Geometry: final body of the model. Coordinates: model frame, mm. Face numbers are marked on the shaded views. A direction names the side the tool comes from. Give positions to 0.01 mm unless a question says otherwise; leave off trailing zeros. Order: outer loops, then holes, each group sorted by start corner. A loop starts at its lowest first (then second) coordinate and runs counter-clockwise, first axis right, second up. Notation, with made-up numbers: (-37.75, 72) - (8.25, 72) arc R29 ccw to (8.25, 98) - close; hole circle Ø11 at (12.25, 2.5). An arc over 180 degrees is marked (long way). Put each result on its own line as item: value. Start each with the question number.
1. Mould query, pull axis X, two halves, no side actions, for the marked faces 3, 4 and 5. Classes: pulls with the +X half, pulls with the -X half, needs draft (parallel to the pull), parting line crosses it, or undercut.
2. Section A-A on x = 3. Return the cut outline in (y, z), plus the area to 3 significant figures.
3. Section D-D on x = -8.25. Return the cut outline in (y, z), plus the area to 3 significant figures.
4. First-contact query: P1, Ø2, axis at x = -5, z = 0, coming from the +Y side; P2, Ø1.6, axis at y = 0.5, z = -2.5, coming from the -X side; P3, Ø0.6, axis at y = 0.5, z = -4, coming from the +X side; P4, Ø1.3, axis at x = -6, z = 1.5, coming from the -Y side. Flat tips, straight axial feed; report the tip coordinate or a pass-through.
5. Ray query, line 1 along Z through (x, y) = (-5, 0.5); line 2 along Y through (x, z) = (3, 4); line 3 along Z through (x, y) = (3.5, 4). Return the intervals inside material, ascending. Write a range as from..to.
6. Set-up query: the marked faces 1 and 2. Return all of +Z, -Z, +X, -X, +Y, -Y with unobstructed straight access to the full face (end or side cutting, diameter ignored); none if empty.
7. Section B-B on z = -5.25. Return the cut outline in (x, y).
8. Section C-C on y = 1.75. Return the cut outline in (x, z).
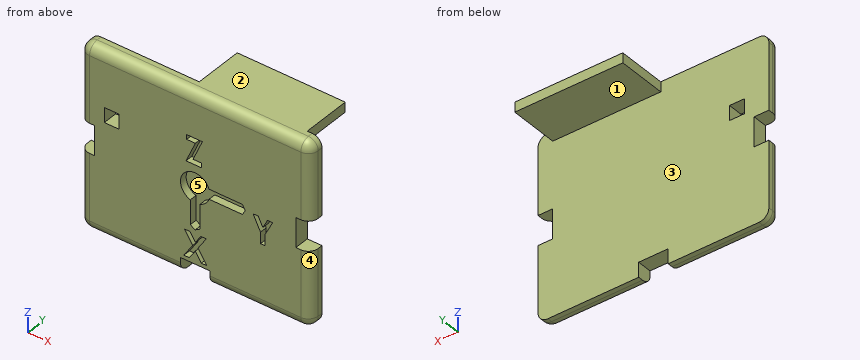
from build123d import *

# Parameters (mm, degrees)
SKETCH1_W           = 23.5
SKETCH1_H           = 18.5
BOSS_EXTRUDE1_DEPTH = 1.5
SKETCH2_W           = 3
SKETCH2_H           = 1.5
SKETCH2_W_2         = 1.5
SKETCH2_H_2         = 3
CUT_EXTRUDE1_DEPTH  = 1.5
SKETCH3_W           = 10
SKETCH3_H           = 1
BOSS_EXTRUDE2_DEPTH = 5
CUT_EXTRUDE3_DEPTH  = 0.75
SKETCH5_W           = 1.5
SKETCH5_H           = 1.5
CUT_EXTRUDE4_DEPTH  = 1.5
FILLET1_R           = 1
FILLET4_R           = 1
SKETCH7_W           = 0.998185699
SKETCH7_H           = 1
BOSS_EXTRUDE3_DEPTH = 5


with BuildPart() as part:
    # Sketch1 → Boss-Extrude1 (new body)
    with BuildSketch(Plane(origin=(0, 0, 0), x_dir=(1, 0, 0), z_dir=(0, 1, 0))):
        with Locations((-5.985849057, 1.668632075)):
            Rectangle(SKETCH1_W, SKETCH1_H)
    extrude(amount=BOSS_EXTRUDE1_DEPTH)

    # Sketch2 → Cut-Extrude1 (cut)
    with BuildSketch(Plane(origin=(0, 1.5, 0), x_dir=(1, 0, 0), z_dir=(0, 1, 0))):
        with Locations((-5.985849057, 10.168632075)):
            Rectangle(SKETCH2_W, SKETCH2_H)
        with Locations((-16.985849057, 1.668632075)):
            Rectangle(SKETCH2_W_2, SKETCH2_H_2)
        with Locations((5.014150943, 1.668632075)):
            Rectangle(SKETCH2_W_2, SKETCH2_H_2)
    extrude(amount=-CUT_EXTRUDE1_DEPTH, mode=Mode.SUBTRACT)

    # Sketch3 → Boss-Extrude2 (add)
    with BuildSketch(Plane(origin=(0, 1.5, 0), x_dir=(1, 0, 0), z_dir=(0, 1, 0))):
        with Locations((-0.735849057, -7.081367925)):
            Rectangle(SKETCH3_W, SKETCH3_H)
    extrude(amount=BOSS_EXTRUDE2_DEPTH)

    # Sketch4 → Cut-Extrude3 (cut)
    with BuildSketch(Plane.XZ):
        with BuildLine():
            Line((-1.177314548, -2.300719994), (-0.888639414, -1.800719994))
            Line((-0.888639414, -1.800719994), (-1.177314548, -1.300719994))
            Line((-1.177314548, -1.300719994), (-4.571635494, -1.300719994))
            ThreePointArc((-4.571635494, -1.300719994), (-7.046509228, -0.740059822), (-6.485849057, -3.214933557))
            Line((-6.485849057, -3.214933557), (-6.485849057, -5.700361827))
            Line((-6.485849057, -5.700361827), (-5.985849057, -5.989036962))
            Line((-5.985849057, -5.989036962), (-5.485849057, -5.700361827))
            Line((-5.485849057, -5.700361827), (-5.485849057, -3.214933557))
            ThreePointArc((-5.485849057, -3.214933557), (-4.925188885, -2.861380166), (-4.571635494, -2.300719994))
            Line((-4.571635494, -2.300719994), (-1.177314548, -2.300719994))
        make_face()
        Polygon((-7.080591406, -6.388557959), (-6.520895893, -6.388557959), (-5.968090572, -7.238171507), (-5.41422522, -6.388557959), (-4.853999693, -6.388557959), (-5.688242815, -7.668013421), (-4.798878165, -9.034391292), (-5.358573678, -9.034391292), (-5.968090572, -8.09732532), (-6.579197509, -9.034391292), (-7.139423037, -9.034391292), (-6.247938328, -7.667483406), align=None)
        Polygon((-6.848224631, 3.131460083), (-5.253940443, 3.131460083), (-6.201606709, 0.960519912), (-5.321782324, 0.960519912), (-5.321782324, 0.48562675), (-6.916066512, 0.48562675), (-5.967870231, 2.656566921), (-6.848224631, 2.656566921), align=None)
        Polygon((-0.096157656, -1.744646719), (0.43226699, -1.744646719), (0.904510079, -2.672702441), (1.376753168, -1.744646719), (1.905177814, -1.744646719), (1.14195666, -3.244588292), (1.14195666, -4.390480052), (0.667063498, -4.390480052), (0.667063498, -3.244588292), align=None)
    extrude(amount=-CUT_EXTRUDE3_DEPTH, mode=Mode.SUBTRACT)

    # Sketch5 → Cut-Extrude4 (cut)
    with BuildSketch(Plane.XZ):
        with Locations((-14.485849057, 1.331367925)):
            Rectangle(SKETCH5_W, SKETCH5_H)
    extrude(amount=-CUT_EXTRUDE4_DEPTH, mode=Mode.SUBTRACT)

    # Fillet1
    fillet1_edges = [part.edges().sort_by_distance(p)[0] for p in [
        (-12.610849057, 0, -10.918632075),
        (5.764150943, 0, -7.043632075),
        (0.639150943, 0, -10.918632075),
        (-17.735849057, 0, -7.043632075),
        (-17.735849057, 0.75, -10.918632075),
        (5.764150943, 0.75, -10.918632075),
    ]]
    fillet(fillet1_edges, radius=FILLET1_R)

    # Fillet4
    fillet4_edges = [part.edges().sort_by_distance(p)[0] for p in [
        (-17.735849057, 0, 3.706367925),
        (5.764150943, 0, 3.706367925),
        (-5.985849057, 0, 7.581367925),
        (5.764150943, 0.75, 7.581367925),
        (-17.735849057, 0.75, 7.581367925),
    ]]
    fillet(fillet4_edges, radius=FILLET4_R)

    # Sketch7 → Boss-Extrude3 (add)
    with BuildSketch(Plane(origin=(0, 1.5, 0), x_dir=(1, 0, 0), z_dir=(0, 1, 0))):
        with Locations((-6.234941907, -7.081367925)):
            Rectangle(SKETCH7_W, SKETCH7_H)
    extrude(amount=BOSS_EXTRUDE3_DEPTH)


solid = part.part
Resolved:
1. face 3: needs draft
1. face 4: pulls with the +X half
1. face 5: undercut
2. outline: (0, -9.92) arc R1 ccw to (1, -10.92) - (1.5, -10.92) - (1.5, 6.58) - (6.5, 6.58) - (6.5, 7.58) - (1, 7.58) arc R1 ccw to (0, 6.58) - close
2. area: 32.3 mm^2
3. outline: (0, -9.92) arc R1 ccw to (1, -10.92) - (1.5, -10.92) - (1.5, 7.58) - (1, 7.58) arc R1 ccw to (0, 6.58) - close
3. area: 27.3 mm^2
4. P1: y = 1.5
4. P2: x = -17.73
4. P3: x = 5.74
4. P4: y = 0
5. line 1: -9.42..-9.03, -8.73..-6.61, -6.39..-2.93, -0.67..7.45
5. line 2: 0..1.5
5. line 3: 6.58..7.58
6. face 1: -Z, +X, -X, +Y
6. face 2: +Z, +X, -X, +Y, -Y
7. outline: (-17.74, 1) arc R1 ccw to (-16.74, 0) - (-6.49, 0) - (-6.49, 0.75) - (-5.49, 0.75) - (-5.49, 0) - (4.76, 0) arc R1 ccw to (5.76, 1) - (5.76, 1.5) - (-17.74, 1.5) - close
8. outline: (-6.73, 6.58) - (4.26, 6.58) - (4.26, 7.58) - (-6.73, 7.58) - close
